from build123d import *

# Parameters (mm, degrees)
SKETCH1_R           = 14
BOSS_EXTRUDE1_DEPTH = 3.6
SKETCH2_R           = 4
BOSS_EXTRUDE2_DEPTH = 5.4
SKETCH3_R           = 5.5
BOSS_EXTRUDE3_DEPTH = 17
SKETCH4_R           = 3.5
CUT_EXTRUDE1_DEPTH  = 17
SKETCH5_R           = 1.75
CUT_EXTRUDE2_DEPTH  = 27.095976701
CIRPATTERN1_COUNT   = 4
SKETCH6_R           = 1.75
CUT_EXTRUDE3_DEPTH  = 27.095976701
FILLET1_R           = 0.5
FILLET2_SIZE        = 0.2


with BuildPart() as part:
    # Sketch1 → Boss-Extrude1 (new body)
    with BuildSketch(Plane.XY):
        Circle(SKETCH1_R)
    extrude(amount=BOSS_EXTRUDE1_DEPTH)

    # Sketch2 → Boss-Extrude2 (add)
    with BuildSketch(Plane.XY.offset(3.6)):
        with Locations(Location((0, 0, 0), (0, 0, 180))):
            Circle(SKETCH2_R)
    extrude(amount=BOSS_EXTRUDE2_DEPTH)

    # Sketch3 → Boss-Extrude3 (add)
    with BuildSketch(Plane(origin=(0, 0, 0), x_dir=(-1, 0, 0), z_dir=(0, 0, -1))):
        Circle(SKETCH3_R)
    extrude(amount=BOSS_EXTRUDE3_DEPTH)

    # Sketch4 → Cut-Extrude1 (cut)
    with BuildSketch(Plane(origin=(0, 0, -17), x_dir=(-1, 0, 0), z_dir=(0, 0, -1))):
        Circle(SKETCH4_R)
    extrude(amount=-CUT_EXTRUDE1_DEPTH, mode=Mode.SUBTRACT)

    # Sketch5 → Cut-Extrude2 (cut, through all)
    with BuildSketch(Plane(origin=(0, 0, 0), x_dir=(-1, 0, 0), z_dir=(0, 0, -1))):
        with Locations((0, 9)):
            Circle(SKETCH5_R)
    cut_extrude2 = extrude(amount=-CUT_EXTRUDE2_DEPTH, mode=Mode.SUBTRACT)

    # CirPattern1: Cut-Extrude2 ×4 about axis
    cirpattern1_axis = Axis((0, 0, 0), (0, 0, 1))
    for i in range(1, CIRPATTERN1_COUNT):
        add(cut_extrude2.rotate(cirpattern1_axis, i * 360 / CIRPATTERN1_COUNT), mode=Mode.SUBTRACT)

    # Sketch6 → Cut-Extrude3 (cut, through all)
    with BuildSketch(Plane(origin=(0, 0, 0), x_dir=(1, 0, 0), z_dir=(0, 1, 0))):
        with Locations(Location((0, 11, 0), (0, 0, 270))):
            Circle(SKETCH6_R)
    extrude(amount=-CUT_EXTRUDE3_DEPTH, mode=Mode.SUBTRACT)

    # Fillet1
    fillet1_edges = [part.edges().sort_by_distance(p)[0] for p in [
        (5.5, 0, -17),
        (4, 0, 9),
    ]]
    fillet(fillet1_edges, radius=FILLET1_R)

    # Fillet2
    fillet2_edges = [part.edges().sort_by_distance(p)[0] for p in [
        (-14, 0, 0),
        (-14, 0, 3.6),
    ]]
    chamfer(fillet2_edges, length=FILLET2_SIZE)


solid = part.part
For this review, take the finished solid that the model builds, in its own axes (mm). A direction names the side the tool comes from. Coordinates: 2 decimals unless noted, no trailing zeros. Order: outer loops, then holes, each group sorted by start corner. A loop starts at its lowest first (then second) coordinate and runs counter-clockwise, first axis right, second up. Notation, with made-up numbers: (74.25, -2.75) - (116.25, -2.75) arc R11 cw to (116.25, 5.25) - close; hole circle Ø7 at (-3, 0.25). An arc over 180 degrees is marked (long way). Use one line per item in the form item = value.
Q1. For faces 4 (the flat face through (6, 0, 0)), 5 (the cylindrical face through (-1.06, -4.25, -12.39)), 6 (the flat face through (3, -3, 3.6)), list the 3-axis set-ups (+Z, -Z, +X, -X, +Y, -Y) from which the entire face can be reached by the end or side of a thin tool; tool diameter is ignored.
Checked values:
face_4 = -Z
face_5 = -Y
face_6 = +Z
Q2. For probe 1 along Y at (x, z) = (0, 2.35); probe 2 along Z at (x, y) = (0, -4.3); probe 3 along Z at (x, y) = (-7, -4.25), list the stretches that pass through material, from the lowest coordinate up. Write a range as from..to.
Checked values:
probe_1 = -14..-10.75, -7.25..7.25, 10.75..14
probe_2 = -17..-12.75, -9.25..3.6
probe_3 = 0..3.6
Q3. Consider section D-D (z = -5.5). Give the boundary of the cut face in (x, y), then the cut area to 3 significant figures.
Checked values:
outline = circle Ø11 at (0, 0); hole circle Ø7 at (0, 0)
area = 56.5 mm2
Q4. Draft analysis for pull direction X (two halves, no side actions). For faces 1 (the cylindrical face through (-10.735, 0.228, 1.775)), 2 (the cylindrical face through (0.867, 3.905, 6.016)), 3 (the flat face through (-2.2, -3.3, -17)), state which applies: +X half, -X half, draft (parallel to the pull), parting line (faces both ways), or undercut.
Checked values:
face_1 = undercut
face_2 = parting line
face_3 = draft
Q5. Consider section B-B (z = 2). Give the boundary of the cut face in (x, y), then the cut area to 3 significant figures.
Checked values:
outline = circle Ø28 at (0, 0); hole circle Ø3.5 at (-9, 0); hole circle Ø3.5 at (0, -9); hole circle Ø3.5 at (0, 9); hole circle Ø3.5 at (9, 0)
area = 577 mm2
Q6. For P1, Ø8, axis at x = 4.5, z = 5, coming from the +Y side; P2, Ø4, axis at x = 1, y = 8.5, coming from the -Z side; P3, Ø12, axis at x = 11, z = -1.5, coming from the +Y side; P4, Ø12, axis at x = -5, y = -1, coming from the -Z side, all flat-tipped, find the tip position at first contact; note any pin that passes through.
Checked values:
P1 = 13.98
P2 = 0
P3 = 12.98
P4 = -17
Q7. Consider section A-A (y = 0). Give the number of separate pieces and of enclosed holes in the cut face, then the cut area to 3 significant figures.
Checked values:
separate_pieces = 3
enclosed_holes = 0
area = 187 mm2
